Part model, mm, in its own coordinate system. A direction names the side the tool comes from. Round coordinates to 2 decimals unless told otherwise and drop trailing zeros. Write each loop counter-clockwise with the first axis right and the second up, starting at its lowest first coordinate (ties: lowest second). Pieces come first, ordered by that corner, then holes.
from build123d import *

# Parameters (mm, degrees)
SKETCH2_R           = 1.55
SKETCH2_R_2         = 2.05
BOSS_EXTRUDE1_DEPTH = 12
FILLET1_R           = 2
CUT_EXTRUDE1_START  = -3
SKETCH3_R           = 3
SKETCH3_R_2         = 2.05
CUT_EXTRUDE1_DEPTH  = 3
SKETCH4_R           = 3.7
CUT_EXTRUDE2_DEPTH  = 4.5
CHAMFER1_SIZE       = 2.4
SKETCH5_R           = 2.75
CUT_EXTRUDE3_DEPTH  = 3
BOSS_EXTRUDE2_START = -9
BOSS_EXTRUDE2_DEPTH = 9
FILLET2_R           = 1
BOSS_EXTRUDE3_DEPTH = 9
FILLET4_START       = -1
FILLET4_DEPTH       = 11
FILLET5_R           = 3


with BuildPart() as part:
    # Sketch2 → Boss-Extrude1 (new body)
    with BuildSketch(Plane.XY):
        with BuildLine():
            ThreePointArc((-34.361900506, 79.761980688), (-39.745042243, 80.625629102), (-42.717452598, 76.055193649))
            Line((-42.717452598, 76.055193649), (-40.859246047, 59.183225371))
            ThreePointArc((-40.859246047, 59.183225371), (-44.528699852, 52.393377917), (-51.756139987, 49.685790659))
            Line((-51.756139987, 49.685790659), (-74.256139987, 49.685790659))
            Line((-74.256139987, 49.685790659), (-80.823457728, 53.261259171))
            ThreePointArc((-80.823457728, 53.261259171), (-87.265010513, 51.801013702), (-86.637858855, 45.225863521))
            Line((-86.637858855, 45.225863521), (-38.5, 0))
            ThreePointArc((-38.5, 0), (-32.095751713, 21.262942459), (-15.013624831, 35.451954381))
            Line((-15.013624831, 35.451954381), (-12.409566879, 56.302830298))
            ThreePointArc((-12.409566879, 56.302830298), (-12.469511691, 58.978105921), (-13.900436048, 61.239333138))
            Line((-13.900436048, 61.239333138), (-34.361900506, 79.761980688))
        make_face()
        with Locations((-37.717452598, 76.055193649)):
            Circle(SKETCH2_R, mode=Mode.SUBTRACT)
        with Locations((-19.197703686, 39.030816229)):
            Circle(SKETCH2_R_2, mode=Mode.SUBTRACT)
        with Locations((-43.007240778, 10.171842851)):
            Circle(SKETCH2_R_2, mode=Mode.SUBTRACT)
        with Locations((-48.5, 15)):
            Circle(SKETCH2_R, mode=Mode.SUBTRACT)
        with Locations((-61.282634195, 39.291280842)):
            Circle(SKETCH2_R_2, mode=Mode.SUBTRACT)
        with Locations((-17.255988141, 57.532546099)):
            Circle(SKETCH2_R, mode=Mode.SUBTRACT)
        with Locations((-83.214262364, 48.86989797)):
            Circle(SKETCH2_R, mode=Mode.SUBTRACT)
    extrude(amount=BOSS_EXTRUDE1_DEPTH)

    # Fillet1
    fillet1_edges = [part.edges().sort_by_distance(p)[0] for p in [
        (-38.5, 0, 6),
    ]]
    fillet(fillet1_edges, radius=FILLET1_R)

    # Sketch3 → Cut-Extrude1 (cut)
    with BuildSketch(Plane.XY.offset(12).offset(CUT_EXTRUDE1_START)):
        with BuildLine():
            ThreePointArc((-80.823457728, 53.261259171), (-87.265010513, 51.801013702), (-86.637858855, 45.225863521))
            Line((-86.637858855, 45.225863521), (-41.629914465, 2.94057708))
            ThreePointArc((-41.629914465, 2.94057708), (-39.567390321, 2.522122518), (-38.272304221, 4.180996249))
            ThreePointArc((-38.272304221, 4.180996249), (-30.892001624, 22.976819529), (-15.013624831, 35.451954381))
            Line((-15.013624831, 35.451954381), (-12.409566879, 56.302830298))
            ThreePointArc((-12.409566879, 56.302830298), (-12.469511691, 58.978105921), (-13.900436048, 61.239333138))
            Line((-13.900436048, 61.239333138), (-34.361900506, 79.761980688))
            ThreePointArc((-34.361900506, 79.761980688), (-39.745042243, 80.625629102), (-42.717452598, 76.055193649))
            Line((-42.717452598, 76.055193649), (-40.859246047, 59.183225371))
            ThreePointArc((-40.859246047, 59.183225371), (-44.528699852, 52.393377917), (-51.756139987, 49.685790659))
            Line((-51.756139987, 49.685790659), (-74.256139987, 49.685790659))
            Line((-74.256139987, 49.685790659), (-80.823457728, 53.261259171))
        make_face()
        with Locations((-83.214262364, 48.86989797)):
            Circle(SKETCH3_R, mode=Mode.SUBTRACT)
        with Locations((-48.5, 15)):
            Circle(SKETCH3_R, mode=Mode.SUBTRACT)
        with Locations((-37.717452598, 76.055193649)):
            Circle(SKETCH3_R, mode=Mode.SUBTRACT)
        with Locations((-17.255988141, 57.532546099)):
            Circle(SKETCH3_R, mode=Mode.SUBTRACT)
        with Locations((-19.197703686, 39.030816229)):
            Circle(SKETCH3_R_2, mode=Mode.SUBTRACT)
        with Locations((-61.282634195, 39.291280842)):
            Circle(SKETCH3_R_2, mode=Mode.SUBTRACT)
        with Locations((-43.007240778, 10.171842851)):
            Circle(SKETCH3_R_2, mode=Mode.SUBTRACT)
    extrude(amount=CUT_EXTRUDE1_DEPTH, mode=Mode.SUBTRACT)

    # Sketch4 → Cut-Extrude2 (cut)
    with BuildSketch(Plane.XY.offset(9)):
        with Locations((-19.197703686, 39.030816229)):
            Circle(SKETCH4_R)
        with Locations((-61.282634195, 39.291280842)):
            Circle(SKETCH4_R)
        with Locations((-43.007240778, 10.171842851)):
            Circle(SKETCH4_R)
    extrude(amount=-CUT_EXTRUDE2_DEPTH, mode=Mode.SUBTRACT)

    # Chamfer1
    # the kernel refuses this chamfer: 2.4 mm, written as the material it adds along each edge
    with BuildSketch(Plane(origin=(-19.197703686, 39.030816229, 4.5), x_dir=(1, 0, 0), z_dir=(0, -1, 0))) as chamfer1_piece_1_section:
        Polygon((3.7, CHAMFER1_SIZE), (3.7 - CHAMFER1_SIZE, 0), (3.7, 0), align=None)
    chamfer1_piece_1 = revolve(axis=Axis((-19.197703686, 39.030816229, 4.5), (0, 0, 1)), mode=Mode.PRIVATE)
    chamfer1_piece_1 = chamfer1_piece_1 - Plane(origin=(-19.197703686, 39.030816229, 4.5), x_dir=(1, 0, 0), z_dir=(0, 0, -1)) * Cylinder(2.05, 15, mode=Mode.PRIVATE)
    add(chamfer1_piece_1)
    with BuildSketch(Plane(origin=(-61.282634195, 39.291280842, 4.5), x_dir=(1, 0, 0), z_dir=(0, -1, 0))) as chamfer1_piece_2_section:
        Polygon((3.7, CHAMFER1_SIZE), (3.7 - CHAMFER1_SIZE, 0), (3.7, 0), align=None)
    chamfer1_piece_2 = revolve(axis=Axis((-61.282634195, 39.291280842, 4.5), (0, 0, 1)), mode=Mode.PRIVATE)
    chamfer1_piece_2 = chamfer1_piece_2 - Plane(origin=(-61.282634195, 39.291280842, 4.5), x_dir=(1, 0, 0), z_dir=(0, 0, -1)) * Cylinder(2.05, 15, mode=Mode.PRIVATE)
    add(chamfer1_piece_2)
    with BuildSketch(Plane(origin=(-43.007240778, 10.171842851, 4.5), x_dir=(1, 0, 0), z_dir=(0, -1, 0))) as chamfer1_piece_3_section:
        Polygon((3.7, CHAMFER1_SIZE), (3.7 - CHAMFER1_SIZE, 0), (3.7, 0), align=None)
    chamfer1_piece_3 = revolve(axis=Axis((-43.007240778, 10.171842851, 4.5), (0, 0, 1)), mode=Mode.PRIVATE)
    chamfer1_piece_3 = chamfer1_piece_3 - Plane(origin=(-43.007240778, 10.171842851, 4.5), x_dir=(1, 0, 0), z_dir=(0, 0, -1)) * Cylinder(2.05, 15, mode=Mode.PRIVATE)
    add(chamfer1_piece_3)

    # Sketch5 → Cut-Extrude3 (cut)
    with BuildSketch(Plane(origin=(0, 0, 0), x_dir=(-1, 0, 0), z_dir=(0, 0, -1))):
        with Locations((37.717452598, 76.055193649)):
            Circle(SKETCH5_R)
        with Locations((83.214262364, 48.86989797)):
            Circle(SKETCH5_R)
        with Locations((17.255988141, 57.532546099)):
            Circle(SKETCH5_R)
        with Locations((48.5, 15)):
            Circle(SKETCH5_R)
    extrude(amount=-CUT_EXTRUDE3_DEPTH, mode=Mode.SUBTRACT)

    # Sketch6 → Boss-Extrude2 (add)
    with BuildSketch(Plane.XY.offset(9).offset(BOSS_EXTRUDE2_START)):
        with BuildLine():
            ThreePointArc((-88.214262364, 48.86989797), (-93.517038002, 45.86989797), (-93.357119507, 51.960370492))
            Line((-93.357119507, 51.960370492), (-94.916514756, 54.893838074))
            ThreePointArc((-94.916514756, 54.893838074), (-98.525385911, 48.481477098), (-94.210921521, 42.520963587))
            ThreePointArc((-94.210921521, 42.520963587), (-89.820992141, 42.315677756), (-86.216712067, 44.830193095))
            Line((-86.216712067, 44.830193095), (-86.637858855, 45.225863521))
            ThreePointArc((-86.637858855, 45.225863521), (-87.803270016, 46.884700557), (-88.214262364, 48.86989797))
        make_face()
        with BuildLine():
            ThreePointArc((-86.216712067, 44.830193095), (-89.820992141, 42.315677756), (-94.210921521, 42.520963587))
            Line((-94.210921521, 42.520963587), (-76.234628888, 35.451954381))
            Line((-76.234628888, 35.451954381), (-86.216712067, 44.830193095))
        make_face()
    extrude(amount=BOSS_EXTRUDE2_DEPTH)

    # Fillet2
    fillet2_edges = [part.edges().sort_by_distance(p)[0] for p in [
        (-94.916514756, 54.893838074, 4.5),
    ]]
    fillet(fillet2_edges, radius=FILLET2_R)

    # Sketch7 → Boss-Extrude3 (add)
    with BuildSketch(Plane.XY.offset(9)):
        with BuildLine():
            Line((-20.572652719, 67.279326905), (-17.607223088, 64.594885231))
            Line((-17.607223088, 64.594885231), (-4.185014718, 79.422033388))
            Line((-4.185014718, 79.422033388), (-7.15044435, 82.106475062))
            ThreePointArc((-7.15044435, 82.106475062), (-7.045073866, 79.987773323), (-9.163775605, 79.882402839))
            Line((-9.163775605, 79.882402839), (-9.709129089, 79.279965693))
            ThreePointArc((-9.709129089, 79.279965693), (-9.169608732, 77.864367662), (-10.631753377, 78.260767761))
            Line((-10.631753377, 78.260767761), (-11.722460344, 77.055893469))
            ThreePointArc((-11.722460344, 77.055893469), (-11.182939988, 75.640295438), (-12.645084632, 76.036695537))
            Line((-12.645084632, 76.036695537), (-13.7357916, 74.831821245))
            ThreePointArc((-13.7357916, 74.831821245), (-13.196271243, 73.416223215), (-14.658415888, 73.812623314))
            Line((-14.658415888, 73.812623314), (-15.749122855, 72.607749022))
            ThreePointArc((-15.749122855, 72.607749022), (-15.209602499, 71.192150991), (-16.671747143, 71.58855109))
            Line((-16.671747143, 71.58855109), (-17.762454111, 70.383676798))
            ThreePointArc((-17.762454111, 70.383676798), (-17.222933754, 68.968078767), (-18.685078398, 69.364478866))
            Line((-18.685078398, 69.364478866), (-20.572652719, 67.279326905))
        make_face()
        with BuildLine():
            Line((-16.826160205, 85.72262571), (-16.280806721, 86.325062856))
            ThreePointArc((-16.280806721, 86.325062856), (-16.386177205, 88.443764595), (-14.267475465, 88.54913508))
            Line((-14.267475465, 88.54913508), (-17.232905097, 91.233576753))
            Line((-17.232905097, 91.233576753), (-30.655113466, 76.406428596))
            Line((-30.655113466, 76.406428596), (-27.689683835, 73.721986922))
            Line((-27.689683835, 73.721986922), (-25.802109514, 75.807138884))
            ThreePointArc((-25.802109514, 75.807138884), (-26.341629871, 77.222736915), (-24.879485226, 76.826336815))
            Line((-24.879485226, 76.826336815), (-23.788778259, 78.031211107))
            ThreePointArc((-23.788778259, 78.031211107), (-24.328298615, 79.446809138), (-22.866153971, 79.050409039))
            Line((-22.866153971, 79.050409039), (-21.775447003, 80.255283331))
            ThreePointArc((-21.775447003, 80.255283331), (-22.31496736, 81.670881362), (-20.852822715, 81.274481263))
            Line((-20.852822715, 81.274481263), (-19.762115748, 82.479355555))
            ThreePointArc((-19.762115748, 82.479355555), (-20.301636104, 83.894953585), (-18.83949146, 83.498553486))
            Line((-18.83949146, 83.498553486), (-17.748784492, 84.703427778))
            ThreePointArc((-17.748784492, 84.703427778), (-18.288304849, 86.119025809), (-16.826160205, 85.72262571))
        make_face()
    extrude(amount=-BOSS_EXTRUDE3_DEPTH)

    # Fillet4: read off the stored shape, not the designer's step
    # Fillet4 outline → Fillet4 (cut)
    with BuildSketch(Plane.XY.offset(FILLET4_START)):
        with BuildLine():
            ThreePointArc((-6.670733599, 81.196144833), (-6.565789093, 81.399975343), (-6.338327999, 81.371310433))
            Line((-6.338327999, 81.371310433), (-7.15044435, 82.106475062))
            ThreePointArc((-7.15044435, 82.106475062), (-6.830087034, 81.693731527), (-6.670733599, 81.196144833))
        make_face()
        with BuildLine():
            ThreePointArc((-15.079591816, 89.284299709), (-15.0284993, 89.060805232), (-15.220911217, 88.936154197))
            ThreePointArc((-15.220911217, 88.936154197), (-14.709968629, 88.826958469), (-14.267475465, 88.54913508))
            Line((-14.267475465, 88.54913508), (-15.079591816, 89.284299709))
        make_face()
    extrude(amount=FILLET4_DEPTH, mode=Mode.SUBTRACT)

    # Fillet5
    fillet5_edges = [part.edges().sort_by_distance(p)[0] for p in [
        (-17.607223088, 64.594885231, 4.5),
        (-30.655113466, 76.406428596, 4.5),
    ]]
    fillet(fillet5_edges, radius=FILLET5_R)


solid = part.part
Q1. Saw through at A-A, the plane y = 15. Write the cut outline in (x, z), and give its area (3 significant figures).
Q2. Two-plate mould, pull along Y, no slides. Class faces 6 (the cylindrical face through (-31.06, 22.75, 4.44)), 7 (the flat face through (-41.8, 67.74, 4.44)), 8 (the cylindrical face through (-34.856, 76.956, 10.479)): released by +Y, released by -Y, zero draft, split by the parting line, or undercut.
Q3. Saw through at B-B, the plane x = -48.5. Write the cut outline in (y, z).
Q4. Saw through at C-C, the plane x = -69. Write the cut outline in (y, z).
Q5. Tool access for faces 1 (the flat face through (-10, 73, 5)), 2 (the flat face through (-50, 14, 3)), 3 (the flat face through (-26.76, 74.75, 4.56)), 4 (the flat face through (-77.494, 51.448, 4.437)), 5 (the cylindrical face through (-46.704, 10.335, 7.965)): list every direction of +Z, -Z, +X, -X, +Y, -Y with a clear straight run to the whole face (end or side of a thin tool).
Q6. Wall check: line 1 (X direction, y = 15, z = 7); line 2 (Y direction, x = -27, z = 4.25); line 3 (Z direction, x = -36, y = 64). Give the ranges that are in metal, low to high.
Q7. Drop flat-ended pins along their axis: P1, Ø8, axis at x = -91.71, y = 48.87, coming from the +Z side; P2, Ø3, axis at x = -18.5, z = 3.5, coming from the -Y side; P3, Ø5.5, axis at x = -19.2, y = 39.03, coming from the +Z side. Give the stop position or say it passes through.
Computed:
1. outline: (-54.47, 0) - (-51.25, 0) - (-51.25, 3) - (-50.05, 3) - (-50.05, 12) - (-51.5, 12) - (-51.5, 9) - (-54.47, 9) - close; (-46.95, 3) - (-45.75, 3) - (-45.75, 0) - (-35.46, 0) - (-35.46, 9) - (-45.5, 9) - (-45.5, 12) - (-46.95, 12) - close
1. area: 145 mm2
2. face 6: released by -Y
2. face 7: undercut
2. face 8: split by the parting line
3. outline: (9.4, 0) - (12.25, 0) - (12.25, 3) - (13.45, 3) - (13.45, 12) - (12, 12) - (12, 9) - (9.4, 9) - close; (16.55, 3) - (17.75, 3) - (17.75, 0) - (50.18, 0) - (50.18, 9) - (18, 9) - (18, 12) - (16.55, 12) - close
4. outline: (28.65, 0) - (49.69, 0) - (49.69, 9) - (28.65, 9) - close
5. face 1: +Z, -Z, +X
5. face 2: -Z
5. face 3: +Z, -Z
5. face 4: +Z, -Z, +Y
5. face 5: +Z
6. line 1: x = -54.47 to -50.05, -46.95 to -35.46
6. line 2: y = 27.45 to 73.1, 74.48 to 80.44
6. line 3: z = 0 to 9
7. P1: stops at z = 9
7. P2: stops at y = 32.9
7. P3: stops at z = 5.95
